The model under review builds one solid part; all positions refer to its coordinate system, in mm. Face numbers are marked on the shaded views. A direction names the side the tool comes from. Give positions to 0.01 mm unless a question says otherwise; leave off trailing zeros. Loops run counter-clockwise (first coordinate to the right, second up) from the corner with the lowest first, then second, coordinate; pieces in that order, holes last. Notation, with made-up numbers: (12.5, 81) - (68.5, 81) arc R24 ccw to (68.5, 116) - close; hole circle Ø8 at (-31, 31). An arc over 180 degrees is marked (long way). Return JSON: item names as keys, results as strings. Group by question number.
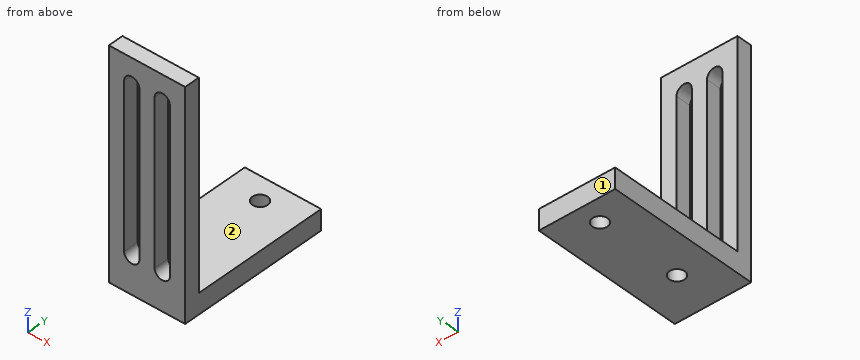
from build123d import *

# Parameters (mm, degrees)
F0_W     = 15
F0_H     = 30
F1_DEPTH = 4
F2_R     = 1.5
F3_DEPTH = 4
F4_W     = 15
F4_H     = 3
F5_DEPTH = 40
F7_DEPTH = 5.334


with BuildPart() as f1:
    # F0 (on Top) → F1 (new body)
    with BuildSketch(Plane.XY):
        with Locations((6.162141, 11.920514)):
            Rectangle(F0_W, F0_H)
    extrude(amount=F1_DEPTH)

    # F2 (on face) → F3 (cut)
    with BuildSketch(Plane.XY.offset(4)):
        with Locations((5.662141, 5.420514)):
            Circle(F2_R)
        with Locations((5.662141, 22.420514)):
            Circle(F2_R)
    extrude(amount=-F3_DEPTH, mode=Mode.SUBTRACT)

    # F4 (on face) → F5 (join)
    with BuildSketch(Plane.XY.offset(4)):
        with Locations((6.162141, -1.579486)):
            Rectangle(F4_W, F4_H)
    extrude(amount=F5_DEPTH)

    # F6 (on face) → F7 (cut)
    with BuildSketch(Plane(origin=(0, -0.079486, 0), x_dir=(-1, 0, 0), z_dir=(0, 1, 0))):
        with BuildLine():
            Line((-10.662141, 39), (-7.662141, 39))
            ThreePointArc((-7.662141, 39), (-9.162141, 40.5), (-10.662141, 39))
        make_face()
        with BuildLine():
            ThreePointArc((-10.662141, 39), (-9.162141, 37.5), (-7.662141, 39))
            Line((-7.662141, 39), (-10.662141, 39))
        make_face()
        with BuildLine():
            Line((-7.662141, 7.299973), (-7.662141, 39))
            ThreePointArc((-7.662141, 39), (-9.162141, 37.5), (-10.662141, 39))
            Line((-10.662141, 39), (-10.662141, 7.299973))
            ThreePointArc((-10.662141, 7.299973), (-9.162141, 8.799973), (-7.662141, 7.299973))
        make_face()
        with BuildLine():
            Line((-10.662141, 7.299973), (-7.662141, 7.299973))
            ThreePointArc((-7.662141, 7.299973), (-9.162141, 8.799973), (-10.662141, 7.299973))
        make_face()
        with BuildLine():
            ThreePointArc((-4.662141, 7.299973), (-3.162141, 5.799973), (-1.662141, 7.299973))
            Line((-1.662141, 7.299973), (-4.662141, 7.299973))
        make_face()
        with BuildLine():
            Line((-4.662141, 7.299973), (-1.662141, 7.299973))
            ThreePointArc((-1.662141, 7.299973), (-3.162141, 8.799973), (-4.662141, 7.299973))
        make_face()
        with BuildLine():
            ThreePointArc((-10.662141, 7.299973), (-9.162141, 5.799973), (-7.662141, 7.299973))
            Line((-7.662141, 7.299973), (-10.662141, 7.299973))
        make_face()
        with BuildLine():
            Line((-1.662141, 7.299973), (-1.662141, 39))
            ThreePointArc((-1.662141, 39), (-3.162141, 37.5), (-4.662141, 39))
            Line((-4.662141, 39), (-4.662141, 7.299973))
            ThreePointArc((-4.662141, 7.299973), (-3.162141, 8.799973), (-1.662141, 7.299973))
        make_face()
        with BuildLine():
            ThreePointArc((-4.662141, 39), (-3.162141, 37.5), (-1.662141, 39))
            Line((-1.662141, 39), (-4.662141, 39))
        make_face()
        with BuildLine():
            Line((-4.662141, 39), (-1.662141, 39))
            ThreePointArc((-1.662141, 39), (-3.162141, 40.5), (-4.662141, 39))
        make_face()
    extrude(amount=-F7_DEPTH, mode=Mode.SUBTRACT)


solid = f1.part
Item 1: For L1, parallel to X at y = -0.75, z = 26; L2, parallel to Z at x = 3.5, y = 15.25; L3, parallel to Y at x = 12, z = 4.5, list the stretches that pass through material, from the lowest coordinate up. Write a range as from..to.
Item 2: Take a section at D-D (x = 0.5). State the section outline as (y, z) points, then the cut area to 3 significant figures.
Item 3: For P1, Ø2.5, axis at x = 5.66, y = 5.42, coming from the -Z side; P2, Ø6, axis at x = 8, z = 32, coming from the +Y side; P3, Ø2, axis at x = 11, y = 19, coming from the -Z side; P4, Ø4, axis at x = 5.66, y = 22.42, coming from the +Z side, all flat-tipped, find the tip position at first contact; note any pin that passes through.
Item 4: Take a section at C-C (y = 6.25). State the section outline as (x, z) points, then the cut area to 3 significant figures.
Item 5: Tool access review of the marked faces 1 and 2: name each direction out of +Z, -Z, +X, -X, +Y, -Y from which nothing blocks a thin tool from reaching the whole face with its end or side.
Item 6: Take a section at A-A (z = 8.5). State the section outline as (x, y) points.
Item 7: Take a section at B-B (x = 5.5). State the section outline as (y, z) points.
Check sheet entries:
{
 "1": {"L1": "x = -1.34..1.66, 4.66..7.66, 10.66..13.66", "L2": "z = 0..4", "L3": "y = -3.08..-0.08"},
 "2": {"outline": "(-3.08, 0) - (26.92, 0) - (26.92, 4) - (-0.08, 4) - (-0.08, 44) - (-3.08, 44) - close", "area": "240 mm^2"},
 "3": {"P1": "passes through", "P2": "stops at y = -0.08", "P3": "stops at z = 0", "P4": "stops at z = 4"},
 "4": {"outline": "(-1.34, 0) - (4.41, 0) - (4.41, 4) - (-1.34, 4) - close; (6.91, 0) - (13.66, 0) - (13.66, 4) - (6.91, 4) - close", "area": "50.0 mm^2"},
 "5": {"face 1": "+Z, -Z, +X, -X, +Y", "face 2": "+Z, +X, -X, +Y"},
 "6": {"outline": "(-1.34, -3.08) - (1.66, -3.08) - (1.66, -0.08) - (-1.34, -0.08) - close; (4.66, -3.08) - (7.66, -3.08) - (7.66, -0.08) - (4.66, -0.08) - close; (10.66, -3.08) - (13.66, -3.08) - (13.66, -0.08) - (10.66, -0.08) - close"},
 "7": {"outline": "(-3.08, 0) - (3.93, 0) - (3.93, 4) - (-0.08, 4) - (-0.08, 44) - (-3.08, 44) - close; (6.91, 0) - (20.93, 0) - (20.93, 4) - (6.91, 4) - close; (23.91, 0) - (26.92, 0) - (26.92, 4) - (23.91, 4) - close"}
}
